```python
from build123d import *

# Parameters (mm, degrees)
SKETCH1_R           = 2.9
BOSS_EXTRUDE1_DEPTH = 1
SKETCH2_W           = 0.25
SKETCH2_H           = 5.8
CUT_EXTRUDE1_DEPTH  = 0.1


with BuildPart() as part:
    # Sketch1 → Boss-Extrude1 (new body)
    with BuildSketch(Plane(origin=(0, 0, 0), x_dir=(1, 0, 0), z_dir=(0, 1, 0))):
        with Locations(Location((-5.348238854, -2.10463103, 0), (0, 0, 270))):
            Circle(SKETCH1_R)
    extrude(amount=BOSS_EXTRUDE1_DEPTH)

    # Sketch2 → Cut-Extrude1 (cut)
    with BuildSketch(Plane(origin=(0, 1, 0), x_dir=(1, 0, 0), z_dir=(0, 1, 0))):
        with Locations((-10.348238854, -2.10463103)):
            Rectangle(SKETCH2_W, SKETCH2_H)
        with Locations((-11.348238854, -2.10463103)):
            Rectangle(SKETCH2_W, SKETCH2_H)
        with Locations((-9.348238854, -2.10463103)):
            Rectangle(SKETCH2_W, SKETCH2_H)
        with Locations((-8.348238854, -2.10463103)):
            Rectangle(SKETCH2_W, SKETCH2_H)
        with Locations((-7.348238854, -2.10463103)):
            Rectangle(SKETCH2_W, SKETCH2_H)
        with Locations((-6.348238854, -2.10463103)):
            Rectangle(SKETCH2_W, SKETCH2_H)
        with Locations((-5.348238854, -2.10463103)):
            Rectangle(SKETCH2_W, SKETCH2_H)
        with Locations((-4.348238854, -2.10463103)):
            Rectangle(SKETCH2_W, SKETCH2_H)
        with Locations((-3.348238854, -2.10463103)):
            Rectangle(SKETCH2_W, SKETCH2_H)
        with Locations((-2.348238854, -2.10463103)):
            Rectangle(SKETCH2_W, SKETCH2_H)
        with Locations((-1.348238854, -2.10463103)):
            Rectangle(SKETCH2_W, SKETCH2_H)
        with Locations((-0.348238854, -2.10463103)):
            Rectangle(SKETCH2_W, SKETCH2_H)
        with Locations((0.651761146, -2.10463103)):
            Rectangle(SKETCH2_W, SKETCH2_H)
        with Locations((1.651761146, -2.10463103)):
            Rectangle(SKETCH2_W, SKETCH2_H)
        with Locations((2.651761146, -2.10463103)):
            Rectangle(SKETCH2_W, SKETCH2_H)
    cut_extrude1 = extrude(amount=-CUT_EXTRUDE1_DEPTH, mode=Mode.SUBTRACT)

    # Mirror1: Cut-Extrude1 across plane
    add(cut_extrude1.mirror(Plane(origin=(0, 0.5, 0), x_dir=(0, 0, 1), z_dir=(0, -1, 0))), mode=Mode.SUBTRACT)


solid = part.part
```
For this review, take the finished solid that the model builds, in its own axes (mm). Round coordinates to 2 decimals unless told otherwise and drop trailing zeros. Write each loop counter-clockwise with the first axis right and the second up, starting at its lowest first coordinate (ties: lowest second). Pieces come first, ordered by that corner, then holes. Notation, with made-up numbers: (38, 49) - (62, 49) arc R27 cw to (62, 76) - close; hole circle Ø3 at (-37, 30). An arc over 180 degrees is marked (long way). Put each result on its own line as item: value.
Q1. We need section C-C (x = -7.7). Give the boundary of the cut face in (y, z), and give its area (3 significant figures).
Solved:
outline: (0, 0.41) - (1, 0.41) - (1, 3.8) - (0, 3.8) - close
area: 3.39 mm2
Q2. We need section A-A (y = 0.25). Give the boundary of the cut face in (x, z).
Solved:
outline: circle Ø5.8 at (-5.35, 2.1)
Q3. We need section B-B (x = -7.1). Give the boundary of the cut face in (y, z), and give its area (3 significant figures).
Solved:
outline: (0, -0.21) - (1, -0.21) - (1, 4.42) - (0, 4.42) - close
area: 4.62 mm2
Q4. Wall thickness on probe 1 along Y at (x, z) = (-3.35, 0.7); probe 2 along X at (y, z) = (0.95, 1.3); probe 3 along Z at (x, y) = (-6.5, 0.45): over which ranges is each line inside the solid? List them lowest first.
Solved:
probe 1: y = 0.1 to 0.9
probe 2: x = -8.13 to -7.47, -7.22 to -6.47, -6.22 to -5.47, -5.22 to -4.47, -4.22 to -3.47, -3.22 to -2.56
probe 3: z = -0.56 to 4.77
